Could you check a few things on this model? Use its own coordinates, in mm. Face numbers are marked on the shaded views. A direction names the side the tool comes from. Coordinates: 2 decimals unless noted, no trailing zeros. Order: outer loops, then holes, each group sorted by start corner. A loop starts at its lowest first (then second) coordinate and runs counter-clockwise, first axis right, second up. Notation, with made-up numbers: (-11, 20) -> (-3, 20) arc R27 ccw to (-3, 46) -> close; hole circle Ø6 at (-25.75, 2). An arc over 180 degrees is marked (long way). Use a Markdown table: item, result. Add a question column.
1) Which directions (+Z, -Z, +X, -X, +Y, -Y) give clear straight access to the entire face, cutting with the end or side of a thin tool? Please do the marked faces 4 and 5.
2) Will these pins go through, and if not, where does the flat tip stop? pin 1 Ø6 at (y, z) = (5, 6.5) entering from +X; pin 2 Ø2 at (x, y) = (8, 11.5) entering from +Z.
3) If we section it at C-C (x = 15): Write out the boundary of the cut face in (y, z), plus the area to 3 significant figures.
4) If we section it at A-A (z = 23): Write out the boundary of the cut face in (x, y).
5) If we section it at B-B (y = 16): Write out the boundary of the cut face in (x, z), plus the area to 3 significant figures.
6) Thinking about a two-plate mould opening in Z: for the marked faces 1, 2 and 3, which applies, +Z half, -Z half, draft (parallel to the pull), parting line (faces both ways), or undercut?
7) If we section it at D-D (x = 55): Write out the boundary of the cut face in (y, z), plus the area to 3 significant figures.
8) If I drill on L1, parallel to X at y = 27.5, z = 24; L2, parallel to X at y = 25, z = 12.5; L3, parallel to Z at x = 23, y = 3, over which ranges is the centre line in solid material (lowest first)? Write a range as [from, to].
```python
from build123d import *

# Parameters (mm, degrees)
F0_W     = 63.5
F0_H     = 63.5
F1_DEPTH = 38.1
F2_R     = 12.7


with BuildPart() as f1:
    # F0 (on Front) → F1 (new body)
    with BuildSketch(Plane.XZ):
        with Locations((31.75, 31.75)):
            Rectangle(F0_W, F0_H)
        with BuildLine():
            ThreePointArc((19.05, 12.7), (13.648367, 15.711607), (13.370387, 21.889806))
            Line((13.370387, 21.889806), (26.070387, 47.289806))
            ThreePointArc((26.070387, 47.289806), (31.75, 50.8), (37.429613, 47.289806))
            Line((37.429613, 47.289806), (50.129613, 21.889806))
            ThreePointArc((50.129613, 21.889806), (49.851633, 15.711607), (44.45, 12.7))
            Line((44.45, 12.7), (19.05, 12.7))
        make_face(mode=Mode.SUBTRACT)
    extrude(amount=-F1_DEPTH)

    # F2
    f2_edges = [f1.edges().sort_by_distance(p)[0] for p in [
        (63.5, 19.05, 63.5),
        (63.5, 19.05, 0),
        (0, 19.05, 63.5),
        (0, 19.05, 0),
    ]]
    fillet(f2_edges, radius=F2_R)


solid = f1.part
```
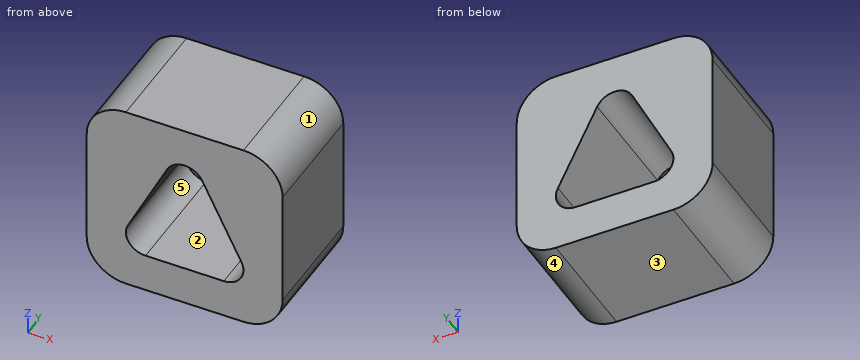
Answer sheet:
| question | item | result |
|---|---|---|
| 1 | face 4 | -Z, +X, +Y, -Y |
| 1 | face 5 | +Y, -Y |
| 2 | pin 1 | x = 63.09 |
| 2 | pin 2 | z = 62.95 |
| 3 | outline | (0, 0) -> (38.1, 0) -> (38.1, 14.16) -> (0, 14.16) -> close; (0, 25.15) -> (38.1, 25.15) -> (38.1, 63.5) -> (0, 63.5) -> close |
| 3 | area | 2,000 mm2 |
| 4 | outline | (0, 0) -> (13.93, 0) -> (13.93, 38.1) -> (0, 38.1) -> close; (49.57, 0) -> (63.5, 0) -> (63.5, 38.1) -> (49.57, 38.1) -> close |
| 5 | outline | (0, 12.7) arc R12.7 ccw to (12.7, 0) -> (50.8, 0) arc R12.7 ccw to (63.5, 12.7) -> (63.5, 50.8) arc R12.7 ccw to (50.8, 63.5) -> (12.7, 63.5) arc R12.7 ccw to (0, 50.8) -> close; hole (13.37, 21.89) arc R6.35 ccw to (19.05, 12.7) -> (44.45, 12.7) arc R6.35 ccw to (50.13, 21.89) -> (37.43, 47.29) arc R6.35 ccw to (26.07, 47.29) -> close |
| 5 | area | 2,920 mm2 |
| 6 | face 1 | +Z half |
| 6 | face 2 | undercut |
| 6 | face 3 | -Z half |
| 7 | outline | (0, 0.71) -> (38.1, 0.71) -> (38.1, 62.79) -> (0, 62.79) -> close |
| 7 | area | 2,360 mm2 |
| 8 | L1 | [0, 14.43], [49.07, 63.5] |
| 8 | L2 | [0, 63.5] |
| 8 | L3 | [0, 12.7], [41.15, 63.5] |
